Input: part model. Units: mm. Frame: model coordinates. A direction names the side the tool comes from. Coordinates: 2 decimals unless noted, no trailing zeros. Loops run counter-clockwise (first coordinate to the right, second up) from the corner with the lowest first, then second, coordinate; pieces in that order, holes last. Notation, with made-up numbers: (17, 39) - (59, 39) arc R23 ccw to (59, 47) - close; hole circle Ø9 at (31.5, -20). An arc over 180 degrees is marked (long way). Answer as CSV lines item,"result". Start each with the question number.
```python
from build123d import *

# Parameters (mm, degrees)
F1_DEPTH = 1140
F2_W     = 600
F2_H     = 420
F3_DEPTH = 655
F4_W     = 600
F4_H     = 420
F5_DEPTH = 655


with BuildPart() as f1:
    # F0 (on Front) → F1 (new body, symmetric)
    with BuildSketch(Plane.XZ):
        Polygon((965, 0), (0, 0), (0, -420), (1245, -420), (1245, -210), (965, -210), align=None)
    extrude(amount=F1_DEPTH, both=True)

    # F2 (on face) → F3 (cut)
    with BuildSketch(Plane.XZ.offset(1140)):
        with Locations((300, -210)):
            Rectangle(F2_W, F2_H)
    extrude(amount=-F3_DEPTH, mode=Mode.SUBTRACT)

    # F4 (on face) → F5 (cut)
    with BuildSketch(Plane(origin=(0, 1140, 0), x_dir=(-1, 0, 0), z_dir=(0, 1, 0))):
        with Locations((-300, -210)):
            Rectangle(F4_W, F4_H)
    extrude(amount=-F5_DEPTH, mode=Mode.SUBTRACT)


solid = f1.part
```
Item 1: Section query B-B, the plane y = -591.5. Output: boundary loops of the cut face in (x, z), and give its area (3 significant figures).
Item 2: Material intervals for probe 1 along Y at (x, z) = (325, -379); probe 2 along X at (y, z) = (1008, -337); probe 3 along X at (y, z) = (-382, -142), sorted ascending.
Item 3: Section query D-D, the plane z = -334. Output: boundary loops of the cut face in (x, y), and give its area (3 significant figures).
Item 4: Section query A-A, the plane z = -55. Output: boundary loops of the cut face in (x, y), and give its area (3 significant figures).
Item 5: Set-up query: faces 1 (the flat face through (0, -7, -207)), 2 (the flat face through (600, -817, -213)), 3 (the flat face through (752, -16, -420)), 4 (the flat face through (1107, -16, -210)), 5 (the flat face through (600, 817, -213)). Return all of +Z, -Z, +X, -X, +Y, -Y with unobstructed straight access to the full face (end or side cutting, diameter ignored); none if empty.
Item 6: Contact query for flat-ended pins moving along their axis: P1, Ø12, axis at x = 1009.5, y = -236.5, coming from the +Z side; P2, Ø6, axis at x = 379.5, z = -108, coming from the -Y side; P3, Ø6, axis at y = 615, z = -206, coming from the -X side. Output: stop coordinate, or through.
Item 7: Draft query along Y for faces 6 (the flat face through (596, -16, 0)), 7 (the flat face through (304, 485, -207)), 8 (the flat face through (296, -485, -207)). Return one class per face: pulls with the +Y half, pulls with the -Y half, needs draft (parallel to the pull), parting line crosses it, or undercut.
Item 8: Section query C-C, the plane x = 1071.5. Output: boundary loops of the cut face in (y, z), and give its area (3 significant figures).
Response values:
1,outline,"(600, -420) - (1245, -420) - (1245, -210) - (965, -210) - (965, 0) - (600, 0) - close"
1,area,"212,000 mm²"
2,probe 1,"y = -485 to 485"
2,probe 2,"x = 600 to 1245"
2,probe 3,"x = 0 to 965"
3,outline,"(0, -485) - (600, -485) - (600, -1140) - (1245, -1140) - (1245, 1140) - (600, 1140) - (600, 485) - (0, 485) - close"
3,area,"2,050,000 mm²"
4,outline,"(0, -485) - (600, -485) - (600, -1140) - (965, -1140) - (965, 1140) - (600, 1140) - (600, 485) - (0, 485) - close"
4,area,"1,410,000 mm²"
5,face 1,"+Z, -Z, -X, +Y, -Y"
5,face 2,"+Z, -Z, -X, -Y"
5,face 3,"-Z, +X, -X, +Y, -Y"
5,face 4,"+Z, +X, +Y, -Y"
5,face 5,"+Z, -Z, -X, +Y"
6,P1,"stops at z = -210"
6,P2,"stops at y = -485"
6,P3,"stops at x = 600"
7,face 6,"needs draft"
7,face 7,"pulls with the +Y half"
7,face 8,"pulls with the -Y half"
8,outline,"(-1140, -420) - (1140, -420) - (1140, -210) - (-1140, -210) - close"
8,area,"479,000 mm²"
